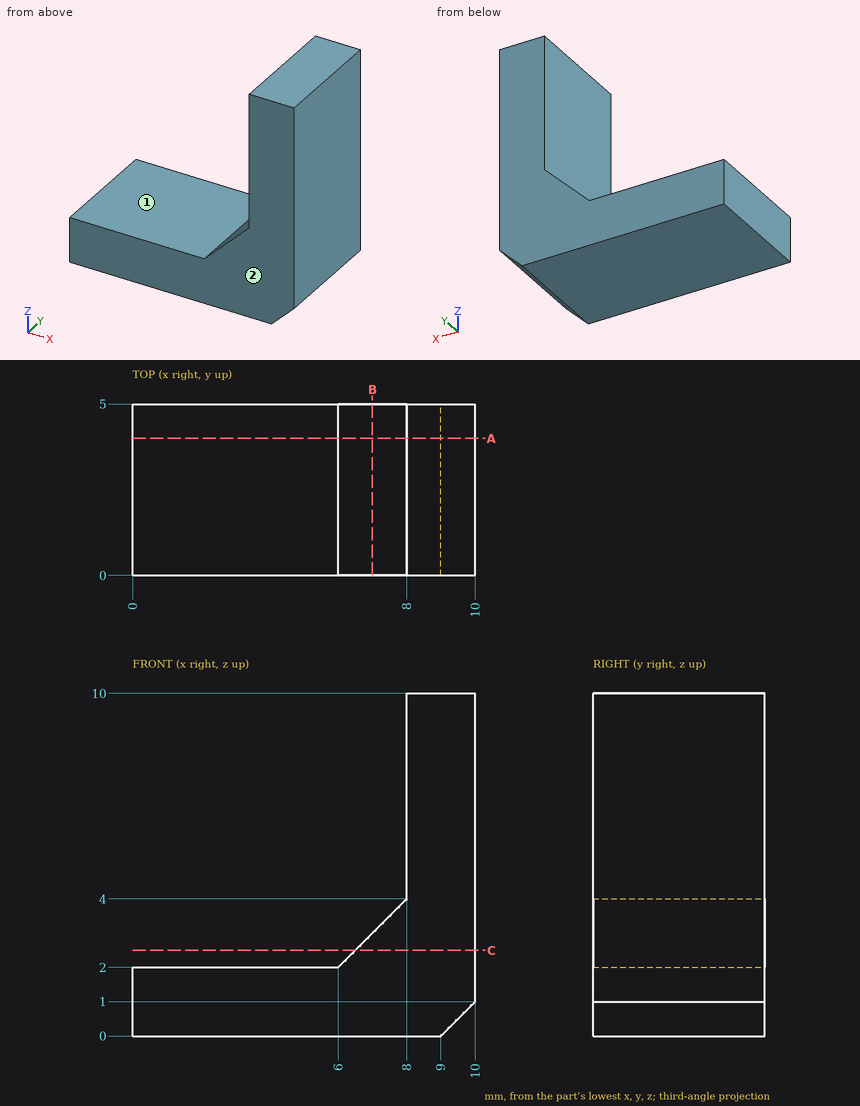
For this review, use the dimensioned drawing (mm, ordinates from the lowest corner) and the shaded views. A direction names the side the tool comes from. Round coordinates to 2 decimals unless told otherwise and drop trailing zeros. Write each loop counter-clockwise with the first axis right and the second up, starting at its lowest first coordinate (ties: lowest second). Pieces come first, ordered by that corner, then holes. Notation, with made-up numbers: (-29.75, 40.25) -> (20.25, 40.25) arc R19 ccw to (20.25, 67.25) -> close; hole circle Ø9 at (11, 38.5). An arc over 180 degrees is marked (long way). Answer in a Markdown table with one row per item.
Q1. Clearance check with flat-ended pins moving along their axes: pin 1 Ø2 at (x, z) = (4, 2.5) entering from +Y; pin 2 Ø1.5 at (x, y) = (1.5, 4) entering from +Z; pin 3 Ø2.5 at (y, z) = (2.5, 6) entering from -X; pin 4 Ø1 at (y, z) = (4.5, 3) entering from -X. State where each tip first meets the part, or that it passes through.
The answers:
| item | result |
|---|---|
| pin 1 | y = 5 |
| pin 2 | z = 2 |
| pin 3 | x = 8 |
| pin 4 | x = 6.5 |
Q2. Take a section at C-C, the plane z = 2.5. State the section outline as (x, y) points, then the cut area to 3 significant figures.
The answers:
| item | result |
|---|---|
| outline | (6.5, 0) -> (10, 0) -> (10, 5) -> (6.5, 5) -> close |
| area | 17.5 mm² |
Q3. For the marked faces 1 and 2, list the 3-axis set-ups (+Z, -Z, +X, -X, +Y, -Y) from which the entire face can be reached by the end or side of a thin tool; tool diameter is ignored.
The answers:
| item | result |
|---|---|
| face 1 | +Z, -X, +Y, -Y |
| face 2 | +Z, -Z, +X, -X, -Y |
Q4. Take a section at B-B, the plane x = 7. State the section outline as (y, z) points, then the cut area to 3 significant figures.
The answers:
| item | result |
|---|---|
| outline | (0, 0) -> (5, 0) -> (5, 3) -> (0, 3) -> close |
| area | 15.0 mm² |
Q5. Take a section at A-A, the plane y = 4. State the section outline as (x, z) points, then the cut area to 3 significant figures.
The answers:
| item | result |
|---|---|
| outline | (0, 0) -> (9, 0) -> (10, 1) -> (10, 10) -> (8, 10) -> (8, 4) -> (6, 2) -> (0, 2) -> close |
| area | 37.5 mm² |
Q6. To check wall thickness, follow L1, parallel to Z at x = 2, y = 0.75; L2, parallel to X at y = 3.2, z = 9.5; L3, parallel to X at y = 0.7, z = 0.75. State the ranges of each line that lie inside material, in increasing order. Write a range as [from, to].
The answers:
| item | result |
|---|---|
| L1 | [0, 2] |
| L2 | [8, 10] |
| L3 | [0, 9.75] |
